Build history of the part. All positions in model axes, mm. Give positions to 0.01 mm unless a question says otherwise; leave off trailing zeros. Order: outer loops, then holes, each group sorted by start corner. A loop starts at its lowest first (then second) coordinate and runs counter-clockwise, first axis right, second up. Notation, with made-up numbers: (62, -39) - (96, -39) arc R14 ccw to (96, -16) - close; hole circle Ø1 at (-36, 53.25). An arc over 180 degrees is marked (long way). One line per item, written item: value.
Autodesk Inventor part; units mm, degrees
ref_plane "Work Plane1" through (-19.1723, 0, 0) normal (0, -0.866, -0.5) x (1, 0, 0)
ref_plane "YZ Plane" through (0, 0, 0) normal (1, 0, 0) x (0, 1, 0)
ref_plane "XZ Plane" through (0, 0, 0) normal (0, 1, 0) x (-1, 0, 0)
sketch "Sketch1" plane through (0, 0, 0) normal (1, 0, 0) x (0, 1, 0)
  line L0 (-9.815, 0) -> (-4.9075, 8.5)
  line L1 (-4.9075, 8.5) -> (4.9075, 8.5)
  line L2 (4.9075, 8.5) -> (9.815, 0)
  line L3 (9.815, 0) -> (4.9075, -8.5)
  line L4 (4.9075, -8.5) -> (-4.9075, -8.5)
  line L5 (-4.9075, -8.5) -> (-9.815, 0)
  point P0 (0, 0)
  point P1 (0, 0)
  dimension "d0" = 19.6299
extrude "Body" add sketch "Sketch1" along normal blind 8
sketch "Sketch2" plane through (0, 0, 0) normal (0, 0, 1) x (1, 0, 0)
  line L0 (0, 4.9075) -> (0, 9.815)
  line L1 (0, 9.815) -> (8, 9.815)
  line L2 (8, 4.9075) -> (8, 9.815)
  line L3 (-1.6, 0) -> (9.6, 0)
  line L4 (1.4809, 9.815) -> (0, 7.25)
  line L5 (6.5191, 9.815) -> (8, 7.25)
  dimension "d3" = 30
  dimension "d4" = 30
  dimension "d5" = 14.5
  dimension "d6" = 14.5
revolve "Chamfer1" cut sketch "Sketch2" angle 360 about axis through (-10, 0, 0) along (1, 0, 0)
sketch "Sketch3" plane through (8, 0, 0) normal (1, 0, 0) x (0, 0, -1)
  arc A0 (-0.625, -1.0825) -> (0.625, -1.0825) centre (0, 0) ccw
hole "Thread" at (8, 0, 0) direction (-1, 0, 0) diameter 8.376 end through all
chamfer "Chamfer2" distance 0.8119 angle 30 1 edges at (8, 0, 4.188) measured on face at (8, 6.1489, -0.7466)
chamfer "Chamfer3" distance 0.8119 angle 30 1 edges at (0, 0, 4.188) measured on face at (0, 6.1489, -0.7466)
ref_plane "Work Plane1" through (-19.1723, 0, 0) normal (0, -0.866, -0.5) x (1, 0, 0)
equation "\"d0\" = 1.1547 * SW"
equation "\"d1\" = KOH"
equation "\"d3\" = ANG1"
equation "\"d4\" = ANG2"
equation "\"d5\" = SW0"
equation "\"d6\" = SW01"
equation "\"d8\" = -0.5 * GD1 + 0.5 * NND"
equation "\"d40\" = -0.5 * GD1 + 0.5 * NND"
equation "\"d10\" = -0.5 * GD1 + 0.5 * NND"
equation "\"d41\" = -0.5 * GD1 + 0.5 * NND"
equation "\"ANG1\" = 30deg"
equation "\"ANG2\" = 30deg"
equation "\"KOH\" = 8"
equation "\"SW\" = 17"
equation "\"SW0\" = 14.5"
equation "\"SW01\" = 14.5"
equation "\"GUL\" = 0.541266 * PTC"
equation "\"TOA\" = 30deg"
equation "\"PTC\" = 1.5"
equation "\"E0\" = 1.155 * SW"
equation "\"GAL\" = 0.541266 * PTC"
properties part number "DIN 555-5 - M10" material "Steel, Mild"
(1) Drill centre lines: line 1 (Z direction, x = 4, y = 0); line 2 (Z direction, x = 7, y = 1.25); line 3 (X direction, y = -8.25, z = -1.5). Where is each one in solid material? Low to high.
Completed:
line 1: -8.5 to -4.19, 4.19 to 8.5
line 2: -8.5 to -4, 4 to 8.5
line 3: 0.66 to 7.34
(2) Slice it at C-C, the plane x = 1. Give the cut face in (y, z), and give its area (3 significant figures).
Completed:
outline: (-8.81, -1.74) - (-5.91, -6.76) arc R8.98 ccw to (-2.9, -8.5) - (2.9, -8.5) arc R8.98 ccw to (5.91, -6.76) - (8.81, -1.74) arc R8.98 ccw to (8.81, 1.74) - (5.91, 6.76) arc R8.98 ccw to (2.9, 8.5) - (-2.9, 8.5) arc R8.98 ccw to (-5.91, 6.76) - (-8.81, 1.74) arc R8.98 ccw to start; hole circle Ø8.38 at (0, 0)
area: 187 mm²
(3) Pin check, flat tips, straight feed: P1, Ø2, axis at x = 2.5, z = 1.5, coming from the +Y side; P2, Ø4, axis at x = 5, z = 6.5, coming from the +Y side; P3, Ø9.5, axis at y = 0, z = 0, coming from the -X side. Stop position of each tip, or through.
Completed:
P1: y = 9.53
P2: y = 7.22
P3: x = 0.14
(4) Pull direction Y, two halves, no side cores. Call faces 1 (the face through (7.907, 6.845, 2.838)), 2 (the face through (3.951, -2.83, 3.087)), 3 (the face through (3.954, 7.327, 4.309)), 4 (the face through (8, -2, -5)): +Y half, -Y half, draft (parallel to the pull), parting line (faces both ways), or undercut.
Completed:
face 1: parting line
face 2: undercut
face 3: +Y half
face 4: draft
(5) Slice it at B-B, the plane y = 0. Give the cut face in (x, z), and give its area (3 significant figures).
Completed:
outline: (0, -7.25) - (0.72, -8.5) - (7.28, -8.5) - (8, -7.25) - (8, -5) - (7.53, -4.19) - (0.47, -4.19) - (0, -5) - close; (0, 5) - (0.47, 4.19) - (7.53, 4.19) - (8, 5) - (8, 7.25) - (7.28, 8.5) - (0.72, 8.5) - (0, 7.25) - close
area: 66.4 mm²
(6) Slice it at A-A, the plane x = 2.75. Give the cut face in (y, z) (1 decimal).
Completed:
outline: (-9.8, 0) - (-4.9, -8.5) - (4.9, -8.5) - (9.8, 0) - (4.9, 8.5) - (-4.9, 8.5) - close; hole circle Ø8.4 at (0, 0)
